from build123d import *

# Parameters (mm, degrees)
BOSS_EXTRUDE1_DEPTH      = 10
BOSS_EXTRUDE1_DEPTH_BACK = 0.01
SKETCH3_W                = 38
SKETCH3_H                = 54
CUT_EXTRUDE1_DEPTH       = 3
SKETCH5_W                = 38
SKETCH5_H                = 54
CUT_EXTRUDE3_DEPTH       = 3
SKETCH7_W                = 165
SKETCH7_H                = 54
CUT_EXTRUDE4_DEPTH       = 6.5
SKETCH9_W                = 19
SKETCH9_H                = 16
SKETCH9_W_2              = 13.23867097
SKETCH9_H_2              = 10.44338859
SKETCH9_W_3              = 14.8958404
SKETCH9_H_3              = 14.23867097
BOSS_EXTRUDE2_DEPTH      = 20.3
SKETCH15_W               = 20
SKETCH15_H               = 50
BOSS_EXTRUDE3_DEPTH      = 20.3
SKETCH16_W               = 7.597238681
SKETCH16_H               = 8
SKETCH16_W_2             = 10
SKETCH16_H_2             = 9.4
SKETCH16_W_3             = 8.7
SKETCH16_H_3             = 8.5
SKETCH16_W_4             = 9.4
SKETCH16_H_4             = 9.3
BOSS_EXTRUDE4_DEPTH      = 30
SKETCH17_R               = 2.55
SKETCH17_R_2             = 3.5
CUT_EXTRUDE17_DEPTH      = 263.983651767
SKETCH18_W               = 43.4
SKETCH18_H               = 43.4
CUT_EXTRUDE18_DEPTH      = 3
SKETCH20_R               = 5
SKETCH20_R_2             = 4
CUT_EXTRUDE20_DEPTH      = 263.983651767
SKETCH21_R               = 9
CUT_EXTRUDE21_DEPTH      = 20
SKETCH22_R               = 1.55
CUT_EXTRUDE23_DEPTH      = 263.010307234
SKETCH25_W               = 8.1
SKETCH25_H               = 59.5
BOSS_EXTRUDE5_DEPTH      = 3.5
SKETCH26_W               = 7.81634734
SKETCH26_H               = 2.399791276
CUT_EXTRUDE24_DEPTH      = 59.5
SKETCH28_W               = 4.75290021
SKETCH28_H               = 9.947843747
BOSS_EXTRUDE6_DEPTH      = 115.870057685
SKETCH30_W               = 14.12
SKETCH30_H               = 25
CUT_EXTRUDE25_DEPTH      = 4.5
SKETCH33_R               = 1.55
CUT_EXTRUDE26_DEPTH      = 10.01
SKETCH36_W               = 38
SKETCH36_H               = 2
BOSS_EXTRUDE7_DEPTH      = 37
SKETCH39_R               = 6
SKETCH39_R_2             = 1.55
CUT_EXTRUDE28_DEPTH      = 2
SKETCH42_R               = 6
SKETCH42_R_2             = 1.55
CUT_EXTRUDE29_DEPTH      = 2


with BuildPart() as part:
    # Sketch1 → Boss-Extrude1 (new, two sides: drawn at the far end of the back side and taken through both)
    with BuildSketch(Plane.XY.offset(-BOSS_EXTRUDE1_DEPTH_BACK)):
        with BuildLine():
            Line((0, 0), (0, -37))
            Line((0, -37), (60, -37))
            Line((60, -37), (60, -52))
            Line((60, -52), (33.129942315, -78.870057685))
            Line((33.129942315, -78.870057685), (-55.850057685, -78.870057685))
            ThreePointArc((-55.850057685, -78.870057685), (-169.614041234, -90.257166815), (-239.999947532, -0.158696229))
            ThreePointArc((-239.999947532, -0.158696229), (-169.748285548, 90.207490359), (-55.850057685, 78.870057685))
            Line((-55.850057685, 78.870057685), (33.129942315, 78.870057685))
            Line((33.129942315, 78.870057685), (60, 52))
            Line((60, 52), (60, 37))
            Line((60, 37), (0, 37))
            Line((0, 37), (0, 0))
        make_face()
    extrude(amount=BOSS_EXTRUDE1_DEPTH + BOSS_EXTRUDE1_DEPTH_BACK)

    # Sketch3 → Cut-Extrude1 (cut)
    with BuildSketch(Plane.XY.offset(10)):
        with Locations((-19, 51.870057685)):
            Rectangle(SKETCH3_W, SKETCH3_H)
    extrude(amount=-CUT_EXTRUDE1_DEPTH, mode=Mode.SUBTRACT)

    # Sketch5 → Cut-Extrude3 (cut)
    with BuildSketch(Plane.XY.offset(10)):
        with Locations((-19, -51.870057685)):
            Rectangle(SKETCH5_W, SKETCH5_H)
    extrude(amount=-CUT_EXTRUDE3_DEPTH, mode=Mode.SUBTRACT)

    # Sketch7 → Cut-Extrude4 (cut)
    with BuildSketch(Plane.XY.offset(10)):
        with Locations((-127.91309413, -21.943838981)):
            Rectangle(SKETCH7_W, SKETCH7_H)
    extrude(amount=-CUT_EXTRUDE4_DEPTH, mode=Mode.SUBTRACT)

    # Sketch9 → Boss-Extrude2 (add)
    with BuildSketch(Plane.XY.offset(10)):
        with Locations((-185.5, 28)):
            Rectangle(SKETCH9_W, SKETCH9_H)
        with Locations((-89.112324575, 12.232539195)):
            Rectangle(SKETCH9_W_2, SKETCH9_H_2)
        with Locations((-124.438795754, -58.044490005)):
            Rectangle(SKETCH9_W_3, SKETCH9_H_3)
    extrude(amount=BOSS_EXTRUDE2_DEPTH)

    # Sketch15 → Boss-Extrude3 (add)
    with BuildSketch(Plane.XY.offset(10)):
        with Locations((-10, 0.20156489)):
            Rectangle(SKETCH15_W, SKETCH15_H)
    extrude(amount=BOSS_EXTRUDE3_DEPTH)

    # Sketch16 → Boss-Extrude4 (add)
    with BuildSketch(Plane.XY.offset(10)):
        with Locations((-228.62215183, 0)):
            Rectangle(SKETCH16_W, SKETCH16_H)
        with Locations((-139.68812176, 89.3492876)):
            Rectangle(SKETCH16_W_2, SKETCH16_H_2)
        with Locations((-66.02791219, 66.09880262)):
            Rectangle(SKETCH16_W_3, SKETCH16_H_3)
        with Locations((-70.67791219, -66.2732878)):
            Rectangle(SKETCH16_W_4, SKETCH16_H_4)
        with Locations((-139.68812176, -88.33151307)):
            Rectangle(SKETCH16_W_2, SKETCH16_H_4)
    extrude(amount=BOSS_EXTRUDE4_DEPTH)

    # Sketch17 → Cut-Extrude17 (cut, through all)
    with BuildSketch(Plane.XY):
        with Locations((-228.42077117, 0)):
            Circle(SKETCH17_R)
        with Locations((-139.68812176, 89.6492876)):
            Circle(SKETCH17_R_2)
        with Locations((-65.87791219, 66.34880262)):
            Circle(SKETCH17_R_2)
        with Locations((-69.87791219, -66.6232878)):
            Circle(SKETCH17_R_2)
        with Locations((-139.68812176, -88.68151307)):
            Circle(SKETCH17_R_2)
    extrude(amount=CUT_EXTRUDE17_DEPTH, mode=Mode.SUBTRACT)

    # Sketch18 → Cut-Extrude18 (cut)
    with BuildSketch(Plane.XY.offset(10)):
        with Locations((-68.42454895, 39.3)):
            Rectangle(SKETCH18_W, SKETCH18_H)
    extrude(amount=-CUT_EXTRUDE18_DEPTH, mode=Mode.SUBTRACT)

    # Sketch20 → Cut-Extrude20 (cut, through all)
    with BuildSketch(Plane.XY):
        with Locations((-185.94705048, 27.1120848)):
            Circle(SKETCH20_R)
        with Locations((-124.709385772, -57.612858016)):
            Circle(SKETCH20_R)
        with Locations((-88.8879152, 12.75038661)):
            Circle(SKETCH20_R_2)
    extrude(amount=CUT_EXTRUDE20_DEPTH, mode=Mode.SUBTRACT)

    # Sketch21 → Cut-Extrude21 (cut)
    with BuildSketch(Plane(origin=(0, 0, 0), x_dir=(0, 0, -1), z_dir=(1, 0, 0))):
        with Locations((-19.36187505, 12.37175029)):
            Circle(SKETCH21_R)
        with Locations((-19.26539558, -14.62824971)):
            Circle(SKETCH21_R)
        with BuildLine():
            Line((-9.491579533, 2.276446619), (-9.557448357, -4.178698144))
            ThreePointArc((-9.557448357, -4.178698144), (-12.081396215, -6.651657156), (-14.554355227, -4.127709299))
            Line((-14.554355227, -4.127709299), (-14.488486403, 2.327435464))
            ThreePointArc((-14.488486403, 2.327435464), (-11.964538545, 4.800394476), (-9.491579533, 2.276446619))
        make_face()
    extrude(amount=-CUT_EXTRUDE21_DEPTH, mode=Mode.SUBTRACT)

    # Sketch22 → Cut-Extrude23 (cut, through all)
    with BuildSketch(Plane.XY.offset(7)):
        with Locations((-88.16862044, 58.97947337)):
            Circle(SKETCH22_R)
        with Locations((-48.76862044, 58.97947337)):
            Circle(SKETCH22_R)
        with Locations((-48.76862044, 19.57947337)):
            Circle(SKETCH22_R)
        with Locations((-88.16862044, 19.57947337)):
            Circle(SKETCH22_R)
    extrude(amount=-CUT_EXTRUDE23_DEPTH, mode=Mode.SUBTRACT)

    # Sketch25 → Boss-Extrude5 (add)
    with BuildSketch(Plane.XY.offset(10)):
        with Locations((-169.64640613, 41.09949177)):
            Rectangle(SKETCH25_W, SKETCH25_H)
    extrude(amount=BOSS_EXTRUDE5_DEPTH)

    # Sketch26 → Cut-Extrude24 (cut)
    with BuildSketch(Plane.XZ.offset(-11.34949177)):
        with Locations((-169.5045798, 11.208428435)):
            Rectangle(SKETCH26_W, SKETCH26_H)
    extrude(amount=-CUT_EXTRUDE24_DEPTH, mode=Mode.SUBTRACT)

    # Sketch28 → Boss-Extrude6 (add)
    with BuildSketch(Plane.XZ.offset(78.870057685)):
        with Locations((16.603067585, 5.033719824)):
            Rectangle(SKETCH28_W, SKETCH28_H)
    extrude(amount=-BOSS_EXTRUDE6_DEPTH)

    # Sketch30 → Cut-Extrude25 (cut)
    with BuildSketch(Plane(origin=(0, 0, -0.01), x_dir=(-1, 0, 0), z_dir=(0, 0, -1))):
        with Locations((-7.06, -49.5)):
            Rectangle(SKETCH30_W, SKETCH30_H)
        Polygon((-14.38072485, 61.935396467), (-14.275539526, 36.935617747), (-0.155664505, 36.995026418), (-0.260849829, 61.994805138), align=None)
    extrude(amount=-CUT_EXTRUDE25_DEPTH, mode=Mode.SUBTRACT)

    # Sketch33 → Cut-Extrude26 (cut)
    with BuildSketch(Plane(origin=(0, 0, -0.01), x_dir=(-1, 0, 0), z_dir=(0, 0, -1))):
        with Locations((-7.06, -53.4)):
            Circle(SKETCH33_R)
        with Locations((-7.06, -49.4)):
            Circle(SKETCH33_R)
        with Locations((-7.06, -45.4)):
            Circle(SKETCH33_R)
        with Locations((-7.06, -41.4)):
            Circle(SKETCH33_R)
        with Locations((-7.228632788, 41.370889137)):
            Circle(SKETCH33_R)
        with Locations((-7.244931474, 45.370855931)):
            Circle(SKETCH33_R)
        with Locations((-7.261230159, 49.370822725)):
            Circle(SKETCH33_R)
        with Locations((-7.277528845, 53.370789519)):
            Circle(SKETCH33_R)
    extrude(amount=-CUT_EXTRUDE26_DEPTH, mode=Mode.SUBTRACT)

    # Sketch36 → Boss-Extrude7 (add)
    with BuildSketch(Plane.XY.offset(7)):
        Polygon((0.279518574, 78.814629504), (0.272425555, 76.814642082), (-37.727335467, 76.949409435), (-37.720242449, 78.949396858), align=None)
        with Locations((-19, -77.815125164)):
            Rectangle(SKETCH36_W, SKETCH36_H)
    extrude(amount=BOSS_EXTRUDE7_DEPTH)

    # Sketch39 → Cut-Extrude28 (cut)
    with BuildSketch(Plane.XZ.offset(78.815125164)):
        with Locations(Location((-19, 19, 0), (0, 0, 270))):
            Circle(SKETCH39_R)
        with Locations(Location((-34.499611559, 25.01055106, 0), (0, 0, 270))):
            Circle(SKETCH39_R_2)
        with Locations(Location((-3.563871147, 24.988758691, 0), (0, 0, 270))):
            Circle(SKETCH39_R_2)
        with Locations(Location((-28.819186805, 37.01055106, 0), (0, 0, 270))):
            Circle(SKETCH39_R_2)
        with Locations(Location((-9.177448314, 36.988758691, 0), (0, 0, 270))):
            Circle(SKETCH39_R_2)
        with Locations(Location((-28.819994175, 13.01055106, 0), (0, 0, 270))):
            Circle(SKETCH39_R_2)
        with Locations(Location((-9.230494356, 12.988758691, 0), (0, 0, 270))):
            Circle(SKETCH39_R_2)
    extrude(amount=-CUT_EXTRUDE28_DEPTH, mode=Mode.SUBTRACT)

    # Sketch42 → Cut-Extrude29 (cut)
    with BuildSketch(Plane(origin=(0.279518574, 78.814629504, 0), x_dir=(0.9999937111161443, -0.003546509292438372, 0), z_dir=(0.003546509292438372, 0.9999937111161443, 0))):
        with Locations(Location((-19.279713392, -19, 0), (0, 0, 180))):
            Circle(SKETCH42_R)
        with Locations(Location((-29.070149337, -13, 0), (0, 0, 180))):
            Circle(SKETCH42_R_2)
        with Locations(Location((-3.778432466, -25, 0), (0, 0, 180))):
            Circle(SKETCH42_R_2)
        with Locations(Location((-9.464104196, -13, 0), (0, 0, 180))):
            Circle(SKETCH42_R_2)
        with Locations(Location((-34.772326096, -25, 0), (0, 0, 180))):
            Circle(SKETCH42_R_2)
        with Locations(Location((-29.096493177, -37, 0), (0, 0, 180))):
            Circle(SKETCH42_R_2)
        with Locations(Location((-9.473371075, -37, 0), (0, 0, 180))):
            Circle(SKETCH42_R_2)
    extrude(amount=-CUT_EXTRUDE29_DEPTH, mode=Mode.SUBTRACT)


solid = part.part
Read the model definition and answer for the solid it produces. Units are mm, in the model's axes. A direction names the side the tool comes from. Give positions to 0.01 mm unless a question says otherwise; leave off trailing zeros. Answer as CSV lines item,"result".
Item 1: For faces 4 (the face through (-131.887, -58, 20)), 5 (the face through (-186, 36, 20)), 6 (the face through (-45.413, -22, 7)), determine the directions among +Z, -Z, +X, -X, +Y, -Y from which every point of the face is accessible in a straight line to the end or side of a thin tool.
Returned:
face 4,"+Z, -X, +Y, -Y"
face 5,"+Z, -X, +Y"
face 6,"+Z"
Item 2: Determine the mould class of faces 1 (the face through (-168.073, -90.903, 4.925)), 2 (the face through (0, -2, 15)), 3 (the face through (-229, 4, 25)) for opening direction X: +X half, -X half, draft (parallel to the pull), parting line (faces both ways), or undercut.
Returned:
face 1,"parting line"
face 2,"undercut"
face 3,"draft"
Item 3: Find section A-A on z = 19. State how many separate pieces and enclosed holes the cut face has, plus the area to 3 significant figures.
Returned:
separate pieces,"15"
enclosed holes,"8"
area,"1,070 mm²"
Item 4: Consider line 1 (Y direction, x = -136, z = 20.5); line 2 (X direction, y = 18.5, z = 3); line 3 (X direction, y = -13, z = 4.5). Determine where each line is inside the solid, lowest interval first. Write a range as [from, to].
Returned:
line 1,"y = [-92.98, -83.68], [84.65, 94.05]"
line 2,"x = [-235.49, -89.28], [-87.06, -49.88], [-47.66, 0], [14.23, 18.98]"
line 3,"x = [-237.2, -210.41], [-45.41, 0], [14.23, 18.98]"
Item 5: Each of these flat-tipped pins is pushed along its axis until it touches: pin 1 (2 mm diameter, centred on x = -140, y = -89, fed in from +Z); pin 2 (7.5 mm diameter, centred on y = 88, z = 25.5, fed in from +X); pin 3 (2.5 mm diameter, centred on y = 55, z = 8.5, fed in from +X). Where does it stop, or does it pass through?
Returned:
pin 1,"stops at z = 0"
pin 2,"stops at x = -134.69"
pin 3,"stops at x = 58.25"
